The model under review builds one solid part; all positions refer to its coordinate system, in mm. Face numbers are marked on the shaded views. A direction names the side the tool comes from. Round coordinates to 2 decimals unless told otherwise and drop trailing zeros. Write each loop counter-clockwise with the first axis right and the second up, starting at its lowest first coordinate (ties: lowest second). Pieces come first, ordered by that corner, then holes. Notation, with made-up numbers: M -18.5,-10 L 24.5,-10 A17 ccw 24.5,6 Z; hole C 5,2.25 d10. An arc over 180 degrees is marked long. Write item = value, one per line. Start each with the question number.
Item 1: Tool access review of the marked faces 1 and 2: name each direction out of +Z, -Z, +X, -X, +Y, -Y from which nothing blocks a thin tool from reaching the whole face with its end or side.
Item 2: Take a section at B-B, the plane y = 3. Give the boundary of the cut face in (x, z).
Item 3: To check wall thickness, follow line 1 along Y through (x, z) = (-0.95, 1.25); line 2 along X through (y, z) = (2, -0.85); line 3 along X through (y, z) = (1, -1.1). State the ranges of each line that lie inside material, in increasing order.
Item 4: For pin 1 Ø1.7 at (x, z) = (0, 0.5) entering from -Y; pin 2 Ø1.5 at (x, y) = (0, -4) entering from +Z; pin 3 Ø1.7 at (x, z) = (1, -0.5) entering from +Y, all flat-tipped, find the tip position at first contact; note any pin that passes through.
Item 5: Take a section at A-A, the plane y = -5.5. Give the boundary of the cut face in (x, z), plus the area to 3 significant figures.
from build123d import *

# Parameters (mm, degrees)
SKETCH2_W           = 3
SKETCH2_H           = 0.5
CUT_EXTRUDE1_DEPTH  = 1.2
FILLET1_R           = 0.1
SKETCH3_R           = 0.2
BOSS_EXTRUDE1_DEPTH = 17.5
SKETCH4_R           = 0.2
BOSS_EXTRUDE2_DEPTH = 1.5


with BuildPart() as part:
    # Sketch1 → Revolve1 (revolve)
    with BuildSketch(Plane.XY):
        with BuildLine():
            Line((0, 0), (0, 5.25))
            Line((0, 5.25), (0.1, 5.25))
            ThreePointArc((0.1, 5.25), (1.089949494, 4.839949494), (1.5, 3.85))
            Line((1.5, 3.85), (1.5, 1.2))
            Line((1.5, 1.2), (1.9, 1.2))
            Line((1.9, 1.2), (1.9, 0))
            Line((1.9, 0), (0, 0))
        make_face()
    revolve(axis=Axis((0, 0, 0), (0, 1, 0)))

    # Sketch2 → Cut-Extrude1 (cut)
    with BuildSketch(Plane(origin=(0, 1.2, 0), x_dir=(1, 0, 0), z_dir=(0, 1, 0))):
        with Locations((0, 1.78)):
            Rectangle(SKETCH2_W, SKETCH2_H)
    extrude(amount=-CUT_EXTRUDE1_DEPTH, mode=Mode.SUBTRACT)

    # Fillet1
    fillet1_edges = [part.edges().sort_by_distance(p)[0] for p in [
        (1.126543386, 0.6, -1.53),
        (-1.126543386, 0.6, -1.53),
        (-1.5, 1.2, 0),
    ]]
    fillet(fillet1_edges, radius=FILLET1_R)

    # Sketch3 → Boss-Extrude1 (add)
    with BuildSketch(Plane.XZ):
        with Locations((0, 1.27)):
            Circle(SKETCH3_R)
        with Locations((0, -1.27)):
            Circle(SKETCH3_R)
    extrude(amount=BOSS_EXTRUDE1_DEPTH)

    # Sketch4 → Boss-Extrude2 (add)
    with BuildSketch(Plane.XZ.offset(17.5)):
        with Locations((0, 1.27)):
            Circle(SKETCH4_R)
    extrude(amount=BOSS_EXTRUDE2_DEPTH)


solid = part.part
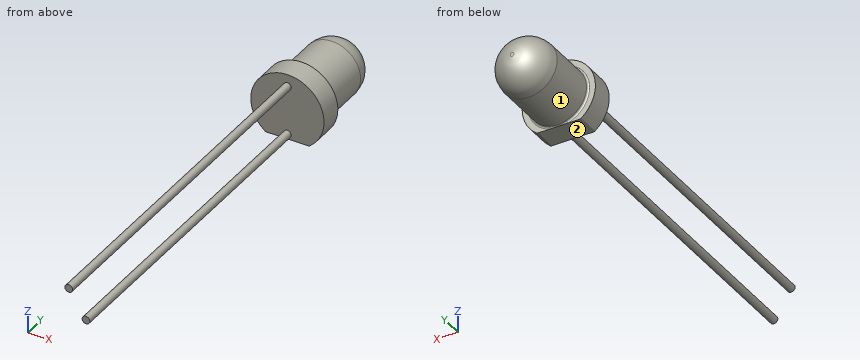
Response values:
q1.face_1 = +Y
q1.face_2 = -Z, +X, -X, +Y, -Y
q2.outline = C 0,0 d3
q3.line_1 = 0 to 1.2
q3.line_2 = -1.24 to 1.24
q3.line_3 = -1.55 to 1.55
q4.pin_1 = -19
q4.pin_2 = 1.47
q4.pin_3 = 5.24
q5.outline = C 0,-1.27 d0.4; C 0,1.27 d0.4
q5.area = 0.251 mm2
